Can you work these out from the model? Positions are in its coordinate system, mm. Face numbers are marked on the shaded views. A direction names the side the tool comes from. Round coordinates to 2 decimals unless told otherwise and drop trailing zeros. Loops run counter-clockwise (first coordinate to the right, second up) from the corner with the lowest first, then second, coordinate; pieces in that order, holes last.
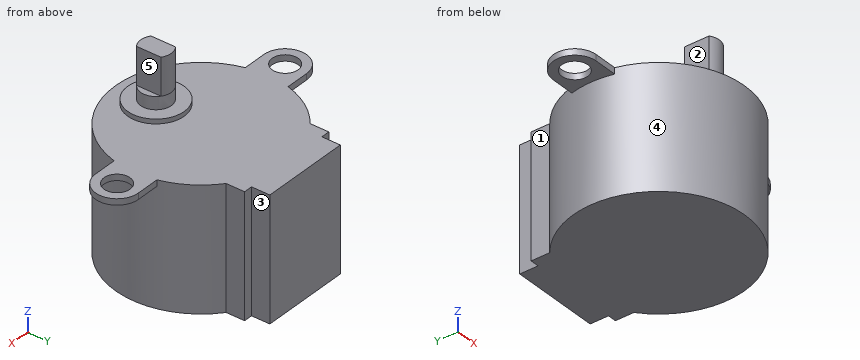
from build123d import *
from build123d.topology import SkipClean

# Parameters (mm, degrees)
EXTRUDE_1_DEPTH = 20
SKETCH_2_R      = 2.125
EXTRUDE_2_DEPTH = 1
SKETCH_3_R      = 4.625
EXTRUDE_3_DEPTH = 0.75
SKETCH_4_R      = 2.5
EXTRUDE_4_DEPTH = 2.05
EXTRUDE_5_DEPTH = 6.05


with BuildPart() as part:
    # Sketch 1 → Extrude 1 (new body)
    with BuildSketch(Plane.XY):
        with BuildLine():
            Line((-7.275, 17), (7.275, 17))
            Line((7.275, 17), (7.275, 14))
            Line((7.275, 14), (8.7, 14))
            Line((8.7, 14), (8.7, 10.968591523))
            ThreePointArc((8.7, 10.968591523), (0, -14), (-8.7, 10.968591523))
            Line((-8.7, 10.968591523), (-8.7, 14))
            Line((-8.7, 14), (-7.275, 14))
            Line((-7.275, 14), (-7.275, 17))
        make_face()
    extrude(amount=EXTRUDE_1_DEPTH)

    # Sketch 2 → Extrude 2 (add)
    with BuildSketch(Plane.XY.offset(20)):
        with BuildLine():
            Line((-17.372355088, 3.5), (17.372355088, 3.5))
            ThreePointArc((17.372355088, 3.5), (20.872355088, 0), (17.372355088, -3.5))
            Line((17.372355088, -3.5), (-17.372355088, -3.5))
            ThreePointArc((-17.372355088, -3.5), (-20.872355088, 0), (-17.372355088, 3.5))
        make_face()
        with Locations((-17.372355088, 0)):
            Circle(SKETCH_2_R, mode=Mode.SUBTRACT)
        with Locations(Location((17.372355088, 0, 0), (0, 0, 180))):
            Circle(SKETCH_2_R, mode=Mode.SUBTRACT)
    extrude(amount=-EXTRUDE_2_DEPTH)

    # Sketch 3 → Extrude 3 (add)
    with BuildSketch(Plane.XY.offset(20)):
        with Locations((0, -7.375)):
            Circle(SKETCH_3_R)
    extrude(amount=EXTRUDE_3_DEPTH)

    # Sketch 4 → Extrude 4 (add)
    with BuildSketch(Plane.XY.offset(20.75)):
        with Locations((0, -7.375)):
            Circle(SKETCH_4_R)
    extrude(amount=EXTRUDE_4_DEPTH)

    # Sketch 5 → Extrude 5 (add)
    with SkipClean():  # the faces are left unmerged after this step: merging them gives an invalid solid
        with BuildSketch(Plane.XY.offset(22.8)):
            with BuildLine():
                Line((-1.5, -9.375), (-1.5, -5.375))
                ThreePointArc((-1.5, -5.375), (0, -4.875), (1.5, -5.375))
                Line((1.5, -5.375), (1.5, -9.375))
                ThreePointArc((1.5, -9.375), (0, -9.875), (-1.5, -9.375))
            make_face()
        extrude(amount=EXTRUDE_5_DEPTH)


solid = part.part
(1) Will these pins go through, and if not, where does the flat tip stop? P1, Ø2, axis at x = 1.5, z = 5, coming from the -Y side; P2, Ø3, axis at x = 16, y = -0.5, coming from the -Z side; P3, Ø1.5, axis at y = 16, z = 13.5, coming from the +X side (3 decimals); P4, Ø2, axis at x = -17, y = -1, coming from the -Z side.
Worked answers:
P1: stops at y = -13.99
P2: stops at z = 19
P3: stops at x = 7.275
P4: passes through
(2) If we section it at C-C, the plane x = -16.5: List the corners of the cut face in (y, z) for me, then the cut area to 3 significant figures.
Worked answers:
outline: (-3.5, 19) - (-1.94, 19) - (-1.94, 20) - (-3.5, 20) - close; (1.94, 19) - (3.5, 19) - (3.5, 20) - (1.94, 20) - close
area: 3.12 mm2
(3) If we section it at A-A, the plane y = 0: List the corners of the cut face in (x, z) for me.
Worked answers:
outline: (-20.87, 19) - (-19.5, 19) - (-19.5, 20) - (-20.87, 20) - close; (-15.25, 19) - (-14, 19) - (-14, 0) - (14, 0) - (14, 19) - (15.25, 19) - (15.25, 20) - (-15.25, 20) - close; (19.5, 19) - (20.87, 19) - (20.87, 20) - (19.5, 20) - close
(4) For the marked faces 1, 2, 3, 4 and 5, which set-ups out of +Z, -Z, +X, -X, +Y, -Y let a thin tool reach every point of the face, with its end or its side?
Worked answers:
face 1: +Z, -Z, -X, +Y
face 2: +Z, -X, +Y, -Y
face 3: +Z, -Z, +X, +Y
face 4: -Z
face 5: +Z, +X, +Y, -Y
(5) If we section it at D-D, the plane x = 0: List the corners of the cut face in (y, z) for me (3 decimals), then the cut area to 3 significant figures.
Worked answers:
outline: (-14, 0) - (17, 0) - (17, 20) - (-2.75, 20) - (-2.75, 20.75) - (-4.875, 20.75) - (-4.875, 28.85) - (-9.875, 28.85) - (-9.875, 20.75) - (-12, 20.75) - (-12, 20) - (-14, 20) - close
area: 667 mm2
(6) If I drill on line 1 (Y direction, x = 0, z = 24) (3 decimals); line 2 (X direction, y = -6, z = 24.25); line 3 (Z direction, x = -16, y = -2.5), over which ranges is the centre line in solid material (lowest first)?
Worked answers:
line 1: y = -9.875 to -4.875
line 2: x = -1.5 to 1.5
line 3: z = 19 to 20
(7) If we section it at B-B, the plane z = 13.75: List the corners of the cut face in (x, y) for me (3 decimals).
Worked answers:
outline: (-8.7, 10.969) arc R14 ccw (long way) to (8.7, 10.969) - (8.7, 14) - (7.275, 14) - (7.275, 17) - (-7.275, 17) - (-7.275, 14) - (-8.7, 14) - close
